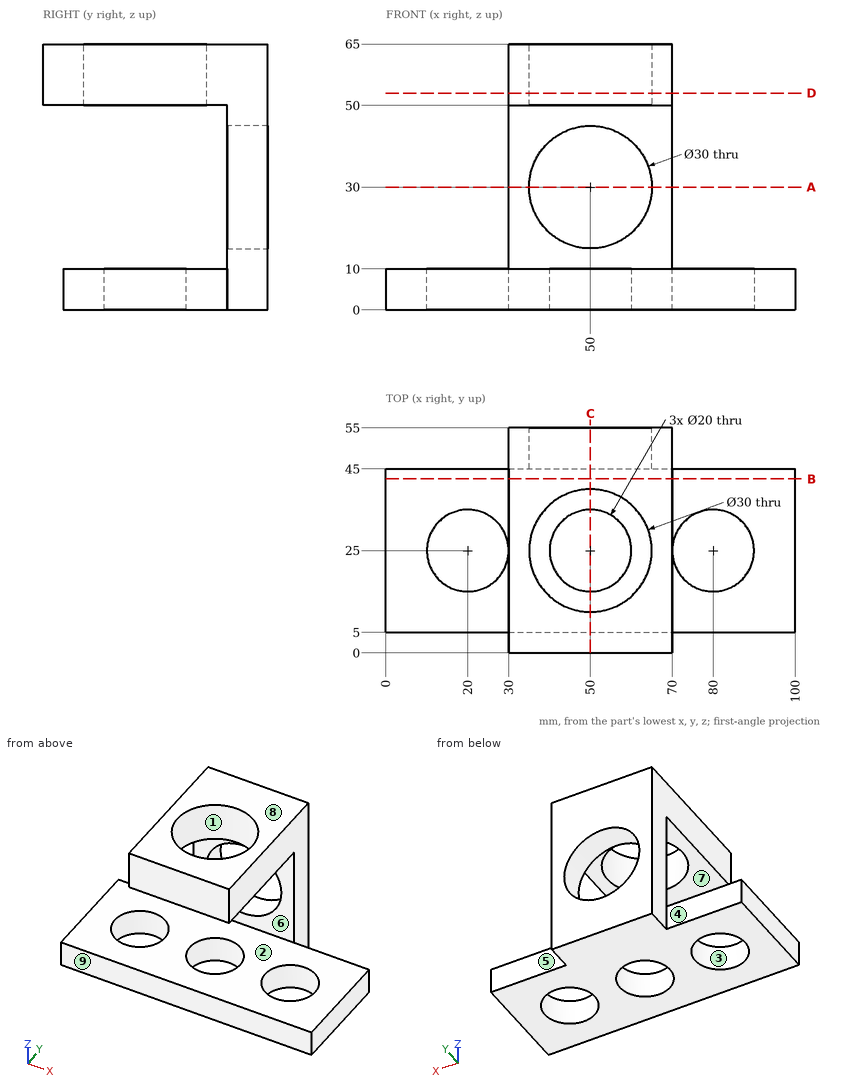
Job drawing, mm, ordinate dimensions from the low corner. One solid piece. A direction names the side the tool comes from. Round coordinates to 2 decimals unless told otherwise and drop trailing zeros. Write each loop counter-clockwise with the first axis right and the second up, starting at its lowest first coordinate (ties: lowest second). Pieces come first, ordered by that corner, then holes.
1) 3-axis set-ups, long thin cutter, end or side, ignore diameter. For the marked faces 1, 2, 3, 4 and 5: which of +Z, -Z, +X, -X, +Y, -Y reach the whole face in a straight line?
2) Band-saw the part on A-A, the plane z = 30. List the corners of the cut face in (x, y).
3) Pin check, flat tips, straight feed: pin 1 (10 mm diameter, centred on y = 34.5, z = 46.5, fed in from +X); pin 2 (5 mm diameter, centred on x = 28.5, z = 7.5, fed in from -Y); pin 3 (2 mm diameter, centred on x = 37, y = 29.5, fed in from -Z); pin 4 (16 mm diameter, centred on x = 80, y = 25, fed in from +Z). Stop position of each tip, or through.
4) Band-saw the part on D-D, the plane z = 53. List the corners of the cut face in (x, y).
5) Drill centre lines: probe 1 along X at (y, z) = (52, 30); probe 2 along Y at (x, z) = (50, 4); probe 3 along Y at (x, z) = (80, 5). Where is each one in solid material? Low to high.
6) Mould opens along Z. For the marked faces 6, 7, 8 and 9 say: +Z half, -Z half, draft (parallel to the pull), parting line (faces both ways), or undercut.
7) Band-saw the part on B-B, the plane y = 42.5. List the corners of the cut face in (x, z), and give its area (3 significant figures).
8) Band-saw the part on C-C, the plane x = 50. List the corners of the cut face in (y, z).
Ans:
1. face 1: +Z
1. face 2: +X, -X, -Y
1. face 3: +Z, -Z
1. face 4: +Z, -Z, -X, +Y
1. face 5: +Z, -Z, +X, +Y
2. outline: (30, 45) - (35, 45) - (35, 55) - (30, 55) - close; (65, 45) - (70, 45) - (70, 55) - (65, 55) - close
3. pin 1: stops at x = 70
3. pin 2: stops at y = 5
3. pin 3: stops at z = 0
3. pin 4: passes through
4. outline: (30, 0) - (70, 0) - (70, 55) - (30, 55) - close; hole circle Ø30 at (50, 25)
5. probe 1: x = 30 to 35, 65 to 70
5. probe 2: y = 5 to 15, 35 to 55
5. probe 3: y = 5 to 15, 35 to 45
6. face 6: undercut
6. face 7: undercut
6. face 8: +Z half
6. face 9: draft
7. outline: (0, 0) - (100, 0) - (100, 10) - (0, 10) - close; (30, 50) - (70, 50) - (70, 65) - (30, 65) - close
7. area: 1,600 mm2
8. outline: (0, 50) - (10, 50) - (10, 65) - (0, 65) - close; (5, 0) - (15, 0) - (15, 10) - (5, 10) - close; (35, 0) - (55, 0) - (55, 15) - (45, 15) - (45, 10) - (35, 10) - close; (40, 50) - (45, 50) - (45, 45) - (55, 45) - (55, 65) - (40, 65) - close
